Geometry check sheet. Reference: drawing and pictorial views, mm from the part's lowest x, y, z. A direction names the side the tool comes from. Round coordinates to 2 decimals unless told otherwise and drop trailing zeros. Write each loop counter-clockwise with the first axis right and the second up, starting at its lowest first coordinate (ties: lowest second). Pieces come first, ordered by that corner, then holes. Notation, with made-up numbers: (77, -2.5) - (115, -2.5) arc R26 ccw to (115, 36.5) - close; hole circle Ø3 at (35.25, -18.75). An arc over 180 degrees is marked (long way). Return JSON: item names as keys, results as strings.
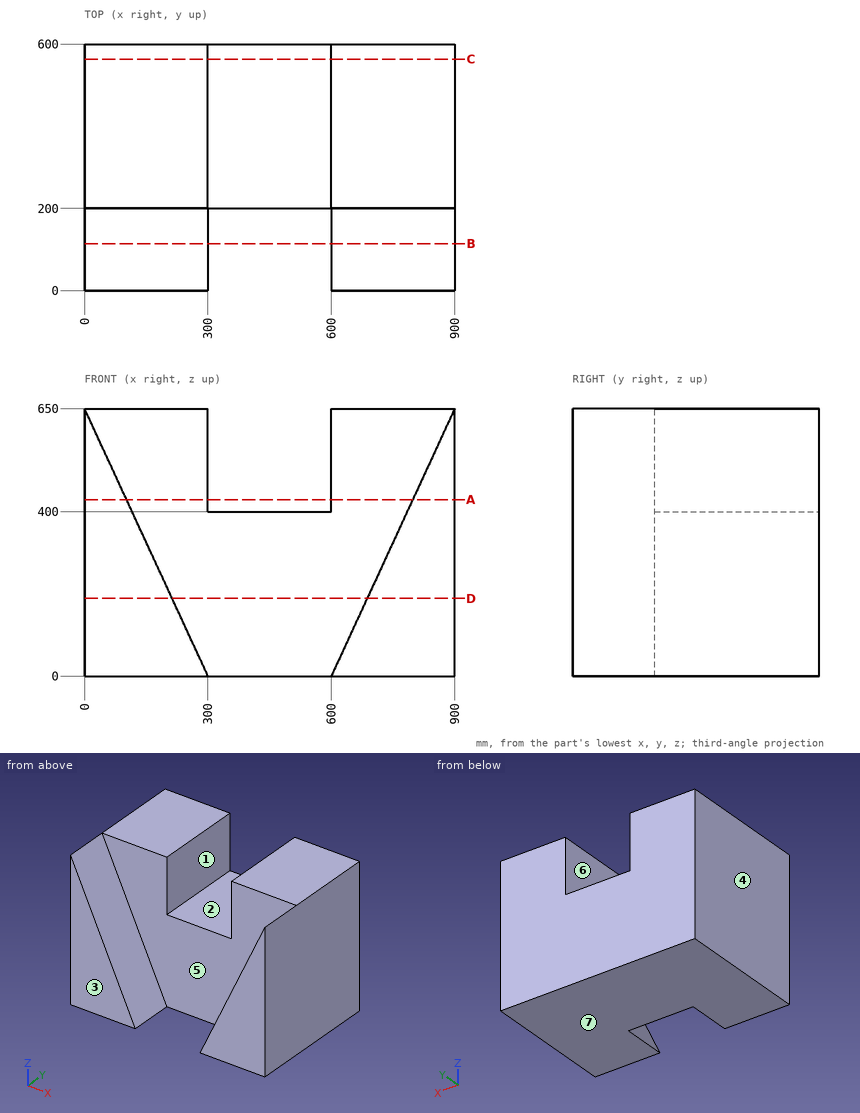
(1) Section check B-B, the plane y = 114.5. Enter the section's corners in (x, z), plus the area to 3 significant figures.
Response values:
{"outline": "(0, 0) - (300, 0) - (0, 650) - close; (600, 0) - (900, 0) - (900, 650) - close", "area": "195,000 mm^2"}
(2) Section check A-A, the plane z = 429. Enter the section's corners in (x, y).
Response values:
{"outline": "(0, 0) - (102, 0) - (102, 200) - (300, 200) - (300, 600) - (0, 600) - close; (600, 200) - (798, 200) - (798, 0) - (900, 0) - (900, 600) - (600, 600) - close"}
(3) Access from +Z, -Z, +X, -X, +Y, -Y to the whole of each face (thin tool, end or side, straight path). Record for the marked faces 5, 6 and 7.
Response values:
{"face 5": "+Z, -Y", "face 6": "+Z, +Y, -Y", "face 7": "-Z, +X, -X, +Y, -Y"}
(4) Release check for a two-part mould opening along X. For the marked faces 1, 2, 3 and 4 record: pulls with the +X half, pulls with the -X half, needs draft (parallel to the pull), parting line crosses it, or undercut.
Response values:
{"face 1": "undercut", "face 2": "undercut", "face 3": "needs draft", "face 4": "pulls with the -X half"}
(5) Section check D-D, the plane z = 188.5. Enter the section's corners in (x, y), plus the area to 3 significant figures.
Response values:
{"outline": "(0, 0) - (213, 0) - (213, 200) - (687, 200) - (687, 0) - (900, 0) - (900, 600) - (0, 600) - close", "area": "445,000 mm^2"}
(6) Material ranges on line 1 along X through (y, z) = (306, 530.5); line 2 along Y through (x, z) = (627, 87.5); line 3 along X through (y, z) = (182, 312.5), recorded low to high. Write a range as [from, to].
Response values:
{"line 1": "x = [0, 300], [600, 900]", "line 2": "y = [200, 600]", "line 3": "x = [0, 155.77], [744.23, 900]"}
(7) Section check C-C, the plane y = 563. Enter the section's corners in (x, z), plus the area to 3 significant figures.
Response values:
{"outline": "(0, 0) - (900, 0) - (900, 650) - (600, 650) - (600, 400) - (300, 400) - (300, 650) - (0, 650) - close", "area": "510,000 mm^2"}
